The listing builds one solid part. Answer for the finished solid, in the listing's coordinates (mm). A direction names the side the tool comes from. Coordinates: 2 decimals unless noted, no trailing zeros. Write each loop counter-clockwise with the first axis right and the second up, starting at its lowest first coordinate (ties: lowest second). Pieces come first, ordered by that corner, then holes. Notation, with made-up numbers: M 12.25,-1.5 L 70.25,-1.5 A11 ccw 70.25,8.5 Z; hole C 43.5,74 d9. An arc over 180 degrees is marked long. Put each result on its own line as item: value. Start each with the question number.
```python
from build123d import *

# Parameters (mm, degrees)
OUTER_START        = 3.175
SKETCH4_R          = 1.143
OUTER_LINK_1_DEPTH = 0.762
SKETCH5_R          = 1.143
PINS_DEPTH         = 3.937


with BuildPart() as part:
    # Sketch4 → outer link 1 (new body)
    with BuildSketch(Plane.XY.offset(OUTER_START)):
        with BuildLine():
            ThreePointArc((-7.224275362, -2.249046818), (-3.937, 0), (-7.224275362, 2.249046818))
            ThreePointArc((-7.224275362, 2.249046818), (-9.525, 1.817591077), (-11.825724638, 2.249046818))
            ThreePointArc((-11.825724638, 2.249046818), (-15.113, 0), (-11.825724638, -2.249046818))
            ThreePointArc((-11.825724638, -2.249046818), (-9.525, -1.817591077), (-7.224275362, -2.249046818))
        make_face()
        with Locations((-12.7, 0)):
            Circle(SKETCH4_R, mode=Mode.SUBTRACT)
        with Locations((-6.35, 0)):
            Circle(SKETCH4_R, mode=Mode.SUBTRACT)
    extrude(amount=-OUTER_LINK_1_DEPTH)


with BuildPart() as body_2:
    # outer link 2: mirrored copy
    add(part.part.mirror(Plane.XY))


with BuildPart() as part_1:
    add(part.part)

    add(body_2.part)  # pins merges body 2
    # Sketch5 → pins (add, symmetric)
    with BuildSketch(Plane.XY):
        with Locations((-12.7, 0)):
            Circle(SKETCH5_R)
        with Locations((-6.35, 0)):
            Circle(SKETCH5_R)
    extrude(amount=PINS_DEPTH, both=True)


solid = part_1.part
```
1) A cutting plane is placed at D-D on y = -1.35. Write down the section's boundary in (x, z) (3 decimals), then the cut area to 3 significant figures.
2) A cutting plane is placed at A-A on x = -6.35. Write down the section's boundary in (y, z) (3 decimals).
3) Given pin 1 Ø1.4 at (x, y) = (-9, 1) entering from +Z (3 decimals); pin 2 Ø1 at (x, y) = (-13.5, 1.5) entering from -Z (3 decimals), each flat-ended and moving along its own axis, determine where each tip first touches the part or whether it passes through.
4) For faces 1 (the face through (-3.94, -0.07, -2.8)), 2 (the face through (-11.644, -0.438, -3.551)), 3 (the face through (-11.644, -0.438, 3.551)), 4 (the face through (-10, 0, 2.413)), 5 (the face through (-6, 0, -3.937)), determine the directions among +Z, -Z, +X, -X, +Y, -Y from which every point of the face is accessible in a straight line to the end or side of a thin tool.
5) A cutting plane is placed at C-C on z = -1.5. Write down the section's boundary in (x, y).
6) Straight lines are drawn through the part: probe 1 along Z at (x, y) = (-14, 1.55) (3 decimals); probe 2 along X at (y, z) = (0.25, 1); probe 3 along X at (y, z) = (-0.3, 3). For each, find the intervals that lie inside material, in ascending order.
7) Determine the mould class of faces 6 (the face through (-10, 0, 3.175)), 7 (the face through (-13, 0, -3.937)), 8 (the face through (-7.49, 0.05, 3.56)) for opening direction X: +X half, -X half, draft (parallel to the pull), parting line (faces both ways), or undercut.
Answers follow:
1. outline: M -14.7,-3.175 L -4.35,-3.175 L -4.35,-2.413 L -14.7,-2.413 Z; M -14.7,2.413 L -4.35,2.413 L -4.35,3.175 L -14.7,3.175 Z
1. area: 15.8 mm²
2. outline: M -2.413,-3.175 L -1.143,-3.175 L -1.143,-3.937 L 1.143,-3.937 L 1.143,-3.175 L 2.413,-3.175 L 2.413,-2.413 L 1.143,-2.413 L 1.143,2.413 L 2.413,2.413 L 2.413,3.175 L 1.143,3.175 L 1.143,3.937 L -1.143,3.937 L -1.143,3.175 L -2.413,3.175 L -2.413,2.413 L -1.143,2.413 L -1.143,-2.413 L -2.413,-2.413 Z
3. pin 1: stops at z = 3.175
3. pin 2: stops at z = -3.175
4. face 1: +Z, -Z
4. face 2: -Z
4. face 3: +Z
4. face 4: none
4. face 5: -Z, +X, -X, +Y, -Y
5. outline: C -12.7,0 d2.29; C -6.35,0 d2.29
6. probe 1: z = -3.175 to -2.413, 2.413 to 3.175
6. probe 2: x = -13.82 to -11.58, -7.47 to -5.23
6. probe 3: x = -15.09 to -3.96
7. face 6: undercut
7. face 7: draft
7. face 8: undercut
